```python
from build123d import *

# Parameters (mm, degrees)
SKETCH_2_W          = 315
SKETCH_2_H          = 15
SKETCH_2_R          = 1.6
EXTRUDE_1_DEPTH     = 15
SKETCH_3_W          = 12
SKETCH_3_H          = 12
CUT_EXTRUDE_1_DEPTH = 316.713477698
SKETCH_4_R          = 1.6
CUT_EXTRUDE_2_DEPTH = 316.713477698


with BuildPart() as part:
    # ｽｹｯﾁ2 → ﾎﾞｽ - 押し出し1 (new body)
    with BuildSketch(Plane.XY):
        with Locations((157.5, -7.5)):
            Rectangle(SKETCH_2_W, SKETCH_2_H)
        with Locations((7.5, -7.5)):
            Circle(SKETCH_2_R, mode=Mode.SUBTRACT)
        with Locations((41.5, -7.5)):
            Circle(SKETCH_2_R, mode=Mode.SUBTRACT)
        with Locations((273.5, -7.5)):
            Circle(SKETCH_2_R, mode=Mode.SUBTRACT)
        with Locations((307.5, -7.5)):
            Circle(SKETCH_2_R, mode=Mode.SUBTRACT)
    extrude(amount=EXTRUDE_1_DEPTH)

    # ｽｹｯﾁ3 → ｶｯﾄ - 押し出し1 (cut, through all)
    with BuildSketch(Plane(origin=(315, 0, 0), x_dir=(0, 0, -1), z_dir=(1, 0, 0))):
        with Locations((-7.5, -7.5)):
            Rectangle(SKETCH_3_W, SKETCH_3_H)
    extrude(amount=-CUT_EXTRUDE_1_DEPTH, mode=Mode.SUBTRACT)

    # ｽｹｯﾁ4 → ｶｯﾄ - 押し出し2 (cut, through all)
    with BuildSketch(Plane(origin=(0, 0, 0), x_dir=(1, 0, 0), z_dir=(0, 1, 0))):
        with Locations(Location((55, -7.5, 0), (0, 0, 270))):
            Circle(SKETCH_4_R)
        with Locations(Location((260, -7.5, 0), (0, 0, 270))):
            Circle(SKETCH_4_R)
    extrude(amount=-CUT_EXTRUDE_2_DEPTH, mode=Mode.SUBTRACT)


solid = part.part
```
CAD build for the part. Positions are in the model's coordinates, mm. A direction names the side the tool comes from. Coordinates: 2 decimals unless noted, no trailing zeros. Order: outer loops, then holes, each group sorted by start corner. A loop starts at its lowest first (then second) coordinate and runs counter-clockwise, first axis right, second up.
(1) Drill centre lines: L1, parallel to X at y = -14.7, z = 7.5; L2, parallel to X at y = -7.5, z = 13.9; L3, parallel to Y at x = 50, z = 3.25. Where is each one in solid material? Low to high.
Solution:
L1: x = 0 to 53.4, 56.6 to 258.4, 261.6 to 315
L2: x = 0 to 5.9, 9.1 to 39.9, 43.1 to 271.9, 275.1 to 305.9, 309.1 to 315
L3: y = -15 to -13.5, -1.5 to 0
(2) Which spindle directions (+Z, -Z, +X, -X, +Y, -Y) get a long thin tool onto all of the face, cutting with end or side? Do faces 4 (the face through (155, -7, 15)), 5 (the face through (160, -1.5, 8)). Say none if no direction does.
Solution:
face 4: +Z, +X, -X, +Y, -Y
face 5: +X, -X
(3) Mould opens along Y. For faces 1 (the face through (160, -8, 13.5)), 2 (the face through (315, -1, 7)), 3 (the face through (155, -15, 7)) say: released by +Y, released by -Y, zero draft, split by the parting line, or undercut.
Solution:
face 1: undercut
face 2: zero draft
face 3: released by -Y
(4) Saw through at A-A, the plane x = 129.5. Write the cut outline in (y, z).
Solution:
outline: (-15, 0) - (0, 0) - (0, 15) - (-15, 15) - close; hole (-13.5, 1.5) - (-1.5, 1.5) - (-1.5, 13.5) - (-13.5, 13.5) - close
(5) Pin check, flat tip, straight feed: pin 1 Ø3 at (x, y) = (307.5, -7.5) entering from +Z. Stop position of the tip, or through.
Solution:
pin 1: passes through
